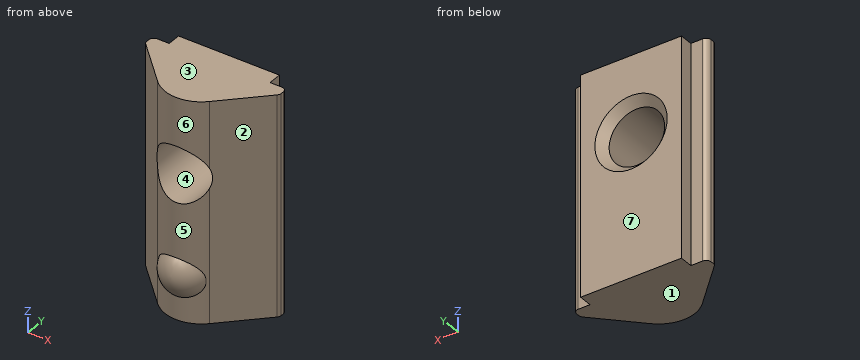
```python
from build123d import *

# Parameters (mm, degrees)
EXTRUDE_1_DEPTH             = 6.5
HOLE_WIZARD_M41_D           = 3.3
HOLE_WIZARD_M41_CSINK_D     = 4.3
HOLE_WIZARD_M41_CSINK_ANGLE = 90
FILLET_1_R                  = 0.3


with BuildPart() as part:
    # Эскиз1 → Бобышка-Вытянуть1 (new body, symmetric)
    with BuildSketch(Plane.XY):
        with BuildLine():
            Line((-3, 0), (3, 0))
            Line((3, 0), (3, -0.8))
            Line((3, -0.8), (4, -0.8))
            Line((4, -0.8), (4, -1.4))
            Line((4, -1.4), (1.536396103, -3.863603897))
            ThreePointArc((1.536396103, -3.863603897), (0, -4.5), (-1.536396103, -3.863603897))
            Line((-1.536396103, -3.863603897), (-4, -1.4))
            Line((-4, -1.4), (-4, -0.8))
            Line((-4, -0.8), (-3, -0.8))
            Line((-3, -0.8), (-3, 0))
        make_face()
    extrude(amount=EXTRUDE_1_DEPTH, both=True)

    # Отверстие обработанное метчиком M41 (through all)
    with Locations(Plane(origin=(0, 0, 0), x_dir=(1, 0, 0), z_dir=(0, 1, 0))):
        with Locations((0, -2)):
            CounterSinkHole(HOLE_WIZARD_M41_D / 2, HOLE_WIZARD_M41_CSINK_D / 2, counter_sink_angle=HOLE_WIZARD_M41_CSINK_ANGLE)

    # Эскиз5 → Повернуть1 (revolve)
    with BuildSketch(Plane(origin=(0, 0, 0), x_dir=(0, 0, -1), z_dir=(1, 0, 0))):
        with BuildLine():
            Line((4, -2), (4, -5))
            ThreePointArc((4, -5), (2.5, -3.5), (4, -2))
        make_face()
    revolve(axis=Axis((0, -2, -4), (0, -1, 0)))

    # Скругление1
    fillet_1_edges = [part.edges().sort_by_distance(p)[0] for p in [
        (4, -0.8, 0),
        (4, -1.4, 0),
        (-4, -1.4, 0),
        (-4, -0.8, 0),
    ]]
    fillet(fillet_1_edges, radius=FILLET_1_R)


solid = part.part
```
Input: part model. Units: mm. Frame: model coordinates. Face numbers are marked on the shaded views. A direction names the side the tool comes from. Give positions to 0.01 mm unless a question says otherwise; leave off trailing zeros. Order: outer loops, then holes, each group sorted by start corner. A loop starts at its lowest first (then second) coordinate and runs counter-clockwise, first axis right, second up. Notation, with made-up numbers: (6.5, 40.25) - (14.5, 40.25) arc R22 cw to (14.5, 69.25) - close; hole circle Ø3 at (14, 18.25). An arc over 180 degrees is marked (long way). Use a Markdown table: item, result.
(1) Access query for the marked faces 5, 6 and 7. Directions: +Z, -Z, +X, -X, +Y, -Y. A direction counts if a zero-diameter tool reaches every point of the face in a straight line with its end or side. Return the directions, or none.
Computed values:
| item | result |
|---|---|
| face 5 | -Y |
| face 6 | +Z, -Y |
| face 7 | +Z, -Z, +X, -X, +Y |
(2) Pin query (flat end, axial travel): pin 1 (1.5 mm diameter, centred on y = -2.5, z = -4.5, fed in from -X); pin 2 (3 mm diameter, centred on x = 0, z = 2, fed in from +Y); pin 3 (3 mm diameter, centred on y = -3, z = 3.5, fed in from +X); pin 4 (1.5 mm diameter, centred on y = -0.5, z = -2, fed in from +X). Return the tip coordinate at first contact, or that it passes through.
Computed values:
| item | result |
|---|---|
| pin 1 | stops at x = -3.65 |
| pin 2 | passes through |
| pin 3 | stops at x = 3.9 |
| pin 4 | stops at x = 4 |
(3) Line query: line 1 (Z direction, x = 0, y = -1.55); line 2 (Y direction, x = 3.25, z = 5.25); line 3 (X direction, y = -1.7, z = -4.25). Output: solid intervals per line, ascending. Write a range as from..to.
Computed values:
| item | result |
|---|---|
| line 1 | z = -6.5..0.35, 3.65..6.5 |
| line 2 | y = -2.15..-0.8 |
| line 3 | x = -3.7..3.7 |
(4) Section query D-D (z = -4.5). Output: boundary loops of the cut face in (x, y).
Computed values:
| item | result |
|---|---|
| outline | (-4, -1.28) arc R0.3 ccw to (-3.91, -1.49) - (-1.54, -3.86) arc R2.17 ccw to (-1.29, -4.07) arc R1.41 ccw to (1.29, -4.07) arc R2.17 ccw to (1.54, -3.86) - (3.91, -1.49) arc R0.3 ccw to (4, -1.28) - (4, -1.1) arc R0.3 ccw to (3.7, -0.8) - (3, -0.8) - (3, 0) - (-3, 0) - (-3, -0.8) - (-3.7, -0.8) arc R0.3 ccw to (-4, -1.1) - close |
(5) Section query A-A (z = 2). Output: boundary loops of the cut face in (x, y).
Computed values:
| item | result |
|---|---|
| outline | (-4, -1.28) arc R0.3 ccw to (-3.91, -1.49) - (-1.65, -3.75) - (-1.65, -0.5) - (-2.15, 0) - (-3, 0) - (-3, -0.8) - (-3.7, -0.8) arc R0.3 ccw to (-4, -1.1) - close; (1.65, -3.75) - (3.91, -1.49) arc R0.3 ccw to (4, -1.28) - (4, -1.1) arc R0.3 ccw to (3.7, -0.8) - (3, -0.8) - (3, 0) - (2.15, 0) - (1.65, -0.5) - close |
(6) Section query C-C (y = -3.3). Output: boundary loops of the cut face in (x, z).
Computed values:
| item | result |
|---|---|
| outline | (-2.1, -6.5) - (2.1, -6.5) - (2.1, 6.5) - (-2.1, 6.5) - close; hole circle Ø3.3 at (0, 2) |
(7) Draft query along Z for the marked faces 1, 2, 3 and 4. Return one class per face: released by +Z, released by -Z, zero draft, split by the parting line, or undercut.
Computed values:
| item | result |
|---|---|
| face 1 | released by -Z |
| face 2 | zero draft |
| face 3 | released by +Z |
| face 4 | undercut |
(8) Section query B-B (x = 0). Output: boundary loops of the cut face in (y, z).
Computed values:
| item | result |
|---|---|
| outline | (-4.5, -6.5) - (0, -6.5) - (0, -0.15) - (-0.5, 0.35) - (-4.5, 0.35) - (-4.5, -2.88) arc R1.5 ccw to (-4.5, -5.12) - close; (-4.5, 3.65) - (-0.5, 3.65) - (0, 4.15) - (0, 6.5) - (-4.5, 6.5) - close |
